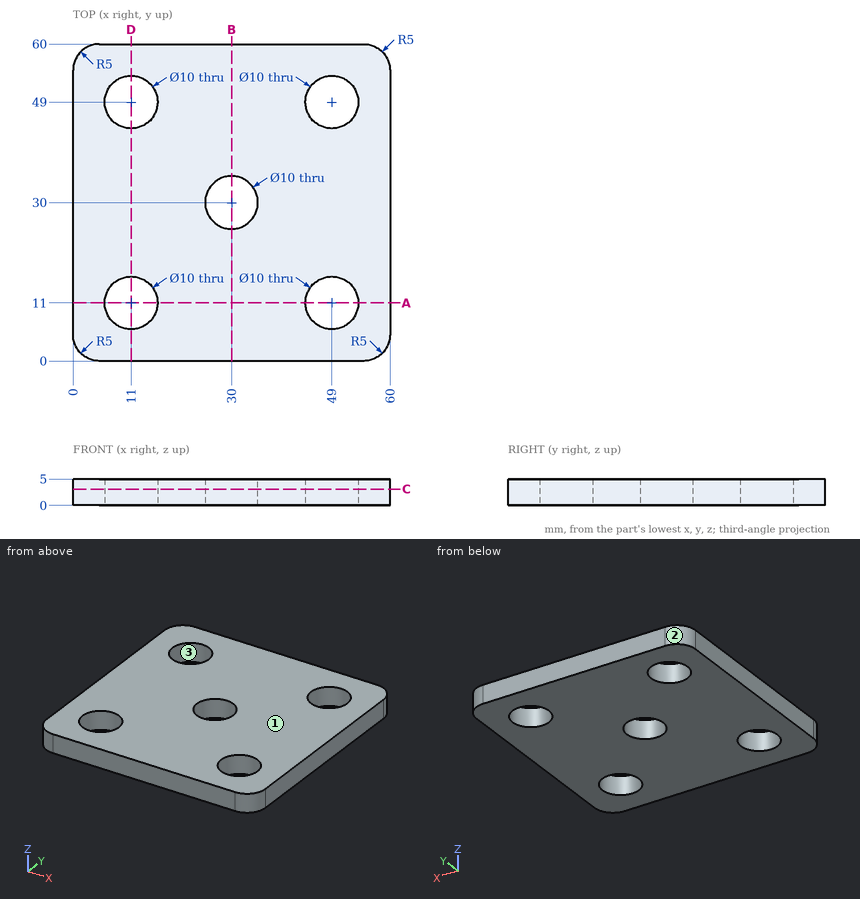
Design review of the part shown in the three views and the two pictorial views. Dimensions are in mm from the part's minimum x, y and z. Give positions to 0.01 mm unless a question says otherwise; leave off trailing zeros. Loops run counter-clockwise (first coordinate to the right, second up) from the corner with the lowest first, then second, coordinate; pieces in that order, holes last. Notation, with made-up numbers: (45.5, 85.25) - (99.5, 85.25) arc R30 cw to (99.5, 121.25) - close; hole circle Ø3 at (-12.75, 19). An arc over 180 degrees is marked (long way). Use CSV: the item, a comma, the result in double quotes. Start each with the question number.
1. Wall thickness on L1, parallel to Y at x = 11, z = 1.75; L2, parallel to X at y = 12.5, z = 0.85: over which ranges is each line inside the solid? List them lowest first.
2. Add section B-B (x = 30). State the section outline as (y, z) points.
3. Add section A-A (y = 11). State the section outline as (x, z) points.
4. Draft analysis for pull direction Y (two halves, no side actions). For the marked faces 1, 2 and 3, state which applies: released by +Y, released by -Y, zero draft, split by the parting line, or undercut.
5. Add section C-C (z = 3.1). State the section outline as (x, y) points, plus the area to 3 significant figures.
Results found:
1,L1,"y = 0 to 6, 16 to 44, 54 to 60"
1,L2,"x = 0 to 6.23, 15.77 to 44.23, 53.77 to 60"
2,outline,"(0, 0) - (25, 0) - (25, 5) - (0, 5) - close; (35, 0) - (60, 0) - (60, 5) - (35, 5) - close"
3,outline,"(0, 0) - (6, 0) - (6, 5) - (0, 5) - close; (16, 0) - (44, 0) - (44, 5) - (16, 5) - close; (54, 0) - (60, 0) - (60, 5) - (54, 5) - close"
4,face 1,"zero draft"
4,face 2,"released by +Y"
4,face 3,"undercut"
5,outline,"(0, 5) arc R5 ccw to (5, 0) - (55, 0) arc R5 ccw to (60, 5) - (60, 55) arc R5 ccw to (55, 60) - (5, 60) arc R5 ccw to (0, 55) - close; hole circle Ø10 at (11, 11); hole circle Ø10 at (11, 49); hole circle Ø10 at (30, 30); hole circle Ø10 at (49, 11); hole circle Ø10 at (49, 49)"
5,area,"3,190 mm²"
